```python
from build123d import *

# Parameters (mm, degrees)
BOSS_EXTRUDE2_DEPTH = 34
CUT_EXTRUDE2_DEPTH  = 32
BOSS_EXTRUDE3_DEPTH = 2
CHAMFER1_SIZE       = 2
CUT_EXTRUDE3_START  = -16.19797
CUT_EXTRUDE3_DEPTH  = 10.135705


with BuildPart() as part:
    # Sketch4 → Boss-Extrude2 (new body)
    with BuildSketch(Plane(origin=(0, 0, 0), x_dir=(1, 0, 0), z_dir=(0, 1, 0))):
        Polygon((-45, 16.197969794), (-45, 8.115066025), (-36.954004115, 3.469708135), (0, -3.046279836), (36.954004115, 3.469708135), (45, 8.115066025), (45, 16.197969794), (38, 12.156517909), (38, 7.537715756), (35.912115049, 6.332274817), (0, 0), (-35.912115049, 6.332274817), (-38, 7.537715756), (-38, 12.156517909), align=None)
    extrude(amount=BOSS_EXTRUDE2_DEPTH)

    # Sketch5 → Cut-Extrude2 (cut)
    with BuildSketch(Plane.XZ):
        Polygon((-40, -8.692416294), (-45, -11.57916764), (-45, -13.888568717), (-40, -11.001817371), align=None)
        Polygon((40, -8.692416294), (45, -11.57916764), (45, -13.888568717), (40, -11.001817371), align=None)
    extrude(amount=-CUT_EXTRUDE2_DEPTH, mode=Mode.SUBTRACT)

    # Sketch6 → Boss-Extrude3 (add)
    with BuildSketch(Plane(origin=(0, 34, 0), x_dir=(1, 0, 0), z_dir=(0, 1, 0))):
        Polygon((38, 12.156517909), (38, 7.537715756), (35.912115049, 6.332274817), (0, 0), (-35.912115049, 6.332274817), (-38, 7.537715756), (-38, 12.156517909), (-29.339745962, 7.156517909), (29.339745962, 7.156517909), align=None)
    extrude(amount=-BOSS_EXTRUDE3_DEPTH)

    # Chamfer1
    chamfer1_edges = [part.edges().sort_by_distance(p)[0] for p in [
        (-40.977002058, 34, -5.79238708),
        (-18.477002058, 34, -0.21171415),
        (18.477002058, 34, -0.21171415),
        (40.977002058, 34, -5.79238708),
    ]]
    chamfer(chamfer1_edges, length=CHAMFER1_SIZE)

    # Sketch7 → Cut-Extrude3 (cut)
    with BuildSketch(Plane.XY.offset(CUT_EXTRUDE3_START)):
        Polygon((-45, 16), (-45, 34), (-41, 34), align=None)
        Polygon((45, 16), (41, 34), (45, 34), align=None)
    extrude(amount=CUT_EXTRUDE3_DEPTH, mode=Mode.SUBTRACT)


solid = part.part
```
For this review, take the finished solid that the model builds, in its own axes (mm). A direction names the side the tool comes from. Coordinates: 2 decimals unless noted, no trailing zeros. Write each loop counter-clockwise with the first axis right and the second up, starting at its lowest first coordinate (ties: lowest second). Pieces come first, ordered by that corner, then holes. Notation, with made-up numbers: (63.5, 0.5) - (85.5, 0.5) arc R13 ccw to (85.5, 9.5) - close; hole circle Ø2 at (-40, 16.5). An arc over 180 degrees is marked (long way). Answer in a Markdown table with one row per item. Add a question column.
Q1. For P1, Ø1, axis at x = -33.5, y = 28, coming from the -Z side; P2, Ø0.7, axis at y = 23.5, z = -10.5, coming from the -X side; P3, Ø2, axis at x = -6.5, y = 33, coming from the -Z side; P4, Ø10, axis at y = 16.5, z = -9, coming from the +X side, all flat-tipped, find the tip position at first contact; note any pin that passes through.
Q2. We need section D-D, the plane y = 12. State the section outline as (x, z) points.
Q3. Tool access review of faces 1 (the flat face through (0, 32, -6)), 2 (the flat face through (-18.74, 15.78, -0.26)), 3 (the flat face through (-42.465, 12.22, -10.116)): name each direction out of +Z, -Z, +X, -X, +Y, -Y from which nothing blocks a thin tool from reaching the whole face with its end or side.
Q4. For probe 1 along Z at (x, y) = (40.5, 22); probe 2 along Y at (x, z) = (16, -3); probe 3 along X at (y, z) = (13, -14.5), list the stretches that pass through material, from the lowest coordinate up.
Q5. We need section A-A, the plane z = -13. State the section outline as (x, y) points, and give its area (3 significant figures).
Q6. We need section B-B, the plane y = 21. State the section outline as (x, z) points, and give its area (3 significant figures).
Q7. We need section C-C, the plane x = -32. State the section outline as (y, z) points, and give its area (3 significant figures).
Q8. Draft analysis for pull direction Z (two halves, no side actions). For faces 4 (the flat face through (36.971, 15.776, -6.943)), 5 (the flat face through (0, 0, 1)), 6 (the flat face through (42.54, 12.22, -12.47)), 7 (the flat face through (38.949, 32.986, -5.76)), state which applies: +Z half, -Z half, draft (parallel to the pull), parting line (faces both ways), or undercut.
Answer list:
| question | item | result |
|---|---|---|
| 1 | P1 | stops at z = -6 |
| 1 | P2 | stops at x = -43.41 |
| 1 | P3 | stops at z = -7.16 |
| 1 | P4 | stops at x = 45 |
| 2 | outline | (-45, -16.2) - (-38, -12.16) - (-38, -7.54) - (-35.91, -6.33) - (0, 0) - (35.91, -6.33) - (38, -7.54) - (38, -12.16) - (45, -16.2) - (45, -13.89) - (40, -11) - (40, -8.69) - (45, -11.58) - (45, -8.12) - (36.95, -3.47) - (0, 3.05) - (-36.95, -3.47) - (-45, -8.12) - (-45, -11.58) - (-40, -8.69) - (-40, -11) - (-45, -13.89) - close |
| 3 | face 1 | -Z, -Y |
| 3 | face 2 | +Z, -X, +Y, -Y |
| 3 | face 3 | -Y |
| 4 | probe 1 | z = -13.6 to -11.29, -8.98 to -5.52 |
| 4 | probe 2 | y = 32 to 34 |
| 4 | probe 3 | x = -45 to -42.06, 42.06 to 45 |
| 5 | outline | (-43.46, 0) - (-39.46, 0) - (-39.46, 34) - (-41, 34) - (-43.46, 22.93) - close; (39.46, 0) - (43.46, 0) - (43.46, 22.93) - (41, 34) - (39.46, 34) - close |
| 5 | area | 245 mm2 |
| 6 | outline | (-43.89, -15.56) - (-38, -12.16) - (-38, -7.54) - (-35.91, -6.33) - (0, 0) - (35.91, -6.33) - (38, -7.54) - (38, -12.16) - (43.89, -15.56) - (43.89, -13.25) - (40, -11) - (40, -8.69) - (43.89, -10.94) - (43.89, -7.47) - (36.95, -3.47) - (0, 3.05) - (-36.95, -3.47) - (-43.89, -7.47) - (-43.89, -10.94) - (-40, -8.69) - (-40, -11) - (-43.89, -13.25) - close |
| 6 | area | 310 mm2 |
| 7 | outline | (0, -5.64) - (32, -5.64) - (32, -8.69) - (34, -8.69) - (34, -4.63) - (32, -2.6) - (0, -2.6) - close |
| 7 | area | 108 mm2 |
| 8 | face 4 | -Z half |
| 8 | face 5 | draft |
| 8 | face 6 | undercut |
| 8 | face 7 | +Z half |
